Input: part model. Units: mm. Frame: model coordinates. A direction names the side the tool comes from. Round coordinates to 2 decimals unless told otherwise and drop trailing zeros. Order: outer loops, then holes, each group sorted by start corner. A loop starts at its lowest first (then second) coordinate and runs counter-clockwise, first axis right, second up. Notation, with made-up numbers: M 54,-14.75 L 101,-14.75 A32 ccw 101,19.25 Z; hole C 54,60 d1. An arc over 180 degrees is marked long. One line per question, with ' | ' between items.
```python
from build123d import *

# Parameters (mm, degrees)
F0_R     = 6.35
F1_DEPTH = 2
F2_DEPTH = 6


with BuildPart() as f1:
    # F0 (on Top) → F1 (new body)
    with BuildSketch(Plane.XY):
        with BuildLine():
            ThreePointArc((-6, 0), (0, -6), (6, 0))
            ThreePointArc((6, 0), (0, 6), (-6, 0))
        make_face()
        with Locations((-300, 0)):
            Circle(F0_R)
        with BuildLine():
            Line((0, 9.35), (-300, 9.35))
            ThreePointArc((-300, 9.35), (-309.35, 0), (-300, -9.35))
            Line((-300, -9.35), (0, -9.349931))
            ThreePointArc((0, -9.349931), (9.349963, 3.5e-05), (0, 9.35))
        make_face()
        with Locations((-300, 0)):
            Circle(F0_R, mode=Mode.SUBTRACT)
        with BuildLine():
            ThreePointArc((-231.35, 0), (-225, 6.35), (-218.65, 0))
            ThreePointArc((-218.65, 0), (-225, -6.35), (-231.35, 0))
        make_face(mode=Mode.SUBTRACT)
        with BuildLine():
            ThreePointArc((-156.35, 0), (-150, 6.35), (-143.65, 0))
            ThreePointArc((-143.65, 0), (-150, -6.35), (-156.35, 0))
        make_face(mode=Mode.SUBTRACT)
        with BuildLine():
            ThreePointArc((-81.35, 0), (-75, 6.35), (-68.65, 0))
            ThreePointArc((-68.65, 0), (-75, -6.35), (-81.35, 0))
        make_face(mode=Mode.SUBTRACT)
        with BuildLine():
            ThreePointArc((-6, 0), (0, 6), (6, 0))
            ThreePointArc((6, 0), (0, -6), (-6, 0))
        make_face(mode=Mode.SUBTRACT)
    extrude(amount=F1_DEPTH)

    # F0 (on Top) → F2 (join)
    with BuildSketch(Plane.XY):
        with BuildLine():
            ThreePointArc((-6, 0), (0, -6), (6, 0))
            ThreePointArc((6, 0), (0, 6), (-6, 0))
        make_face()
    extrude(amount=F2_DEPTH)


solid = f1.part
```
Item 1: First-contact query: pin 1 (1 mm diameter, centred on y = 1.5, z = 0.5, fed in from -X); pin 2 (10 mm diameter, centred on x = -37.5, y = 5.5, fed in from +Z). Flat tips, straight axial feed; report the tip coordinate or a pass-through.
Report:
pin 1: x = -309.3 | pin 2: z = 2
Item 2: Mould query, pull axis Y, two halves, no side actions, for faces 3 (the cylindrical face through (-143.943, -1.907, 0.986)), 4 (the flat face through (-152.2, 6.4, 0)), 5 (the cylindrical face through (9.348, -0.206, 0.986)). Classes: +Y half, -Y half, draft (parallel to the pull), parting line (faces both ways), or undercut.
Report:
face 3: undercut | face 4: draft | face 5: parting line
Item 3: Section query D-D, the plane x = -52. Return loops of the section in (y, z), plus the area to 3 significant figures.
Report:
outline: M -9.35,0 L 9.35,0 L 9.35,2 L -9.35,2 Z | area: 37.4 mm²
Item 4: Line query: line 1 along Y through (x, z) = (-150, 0.9); line 2 along X through (y, z) = (1.5, 1.8); line 3 along Z through (x, y) = (-217, 4). Output: solid intervals per line, ascending. Write a range as from..to.
Report:
line 1: -9.35..-6.35, 6.35..9.35 | line 2: -309.23..-306.17, -293.83..-231.17, -218.83..-156.17, -143.83..-81.17, -68.83..9.23 | line 3: 0..2
Item 5: Access query for faces 1 (the cylindrical face through (-6, 0, 4)), 2 (the cylindrical face through (-306.344, 0.279, 0.986)). Directions: +Z, -Z, +X, -X, +Y, -Y. A direction counts if a zero-diameter tool reaches every point of the face in a straight line with its end or side. Return the directions, or none.
Report:
face 1: +Z | face 2: +Z, -Z
Item 6: Section query C-C, the plane x = -225. Return loops of the section in (y, z), plus the area to 3 significant figures.
Report:
outline: M -9.35,0 L -6.35,0 L -6.35,2 L -9.35,2 Z; M 6.35,0 L 9.35,0 L 9.35,2 L 6.35,2 Z | area: 12.0 mm²
Item 7: Section query A-A, the plane y = 0. Return loops of the section in (x, z), plus the area to 3 significant figures.
Report:
outline: M -309.35,0 L -306.35,0 L -306.35,2 L -309.35,2 Z; M -293.65,0 L -231.35,0 L -231.35,2 L -293.65,2 Z; M -218.65,0 L -156.35,0 L -156.35,2 L -218.65,2 Z; M -143.65,0 L -81.35,0 L -81.35,2 L -143.65,2 Z; M -68.65,0 L 9.35,0 L 9.35,2 L 6,2 L 6,6 L -6,6 L -6,2 L -68.65,2 Z | area: 584 mm²
Item 8: Section query B-B, the plane z = 1.1. Return loops of the section in (x, y).
Report:
outline: M -300,-9.35 L 0,-9.35 A9.35 ccw 0,9.35 L -300,9.35 A9.35 ccw Z; hole C -300,0 d12.7; hole C -225,0 d12.7; hole C -150,0 d12.7; hole C -75,0 d12.7
